Input: part model. Units: mm. Frame: model coordinates. A direction names the side the tool comes from. Give positions to 0.01 mm unless a question says otherwise; leave off trailing zeros. Write each loop counter-clockwise with the first axis right and the second up, starting at its lowest first coordinate (ties: lowest second). Pieces come first, ordered by that corner, then holes. Notation, with made-up numbers: (83, 49.5) -> (136, 49.5) arc R32 ccw to (136, 76.5) -> close; hole circle Ø1 at (-34, 74). An arc over 180 degrees is marked (long way). Answer as a JSON object with one key per item and string values. Group by question number.
from build123d import *

# Parameters (mm, degrees)
F0_R     = 30
F0_W     = 4
F0_H     = 4
F0_R_2   = 1.5
F1_DEPTH = 4
F2_R     = 2.25
F3_DEPTH = 2.6
F4_R     = 19
F4_R_2   = 1.5
F5_DEPTH = 0.1


with BuildPart() as f1:
    # F0 (on Top) → F1 (new body)
    with BuildSketch(Plane.XY):
        Circle(F0_R)
        with Locations((-26, 0)):
            Rectangle(F0_W, F0_H, mode=Mode.SUBTRACT)
        Circle(F0_R_2, mode=Mode.SUBTRACT)
        with Locations((26, 0)):
            Rectangle(F0_W, F0_H, mode=Mode.SUBTRACT)
    extrude(amount=F1_DEPTH)

    # F2 (on face) → F3 (cut)
    with BuildSketch(Plane.XY.offset(4)):
        with Locations((-18.197132, 18.083166)):
            Circle(F2_R)
        with Locations((18.083166, 18.197132)):
            Circle(F2_R)
        with Locations((-18.083166, -18.197132)):
            Circle(F2_R)
        with Locations((18.197132, -18.083166)):
            Circle(F2_R)
    extrude(amount=-F3_DEPTH, mode=Mode.SUBTRACT)

    # F4 (on face) → F5 (cut)
    with BuildSketch(Plane.XY.offset(4)):
        Circle(F4_R)
        Circle(F4_R_2, mode=Mode.SUBTRACT)
    extrude(amount=-F5_DEPTH, mode=Mode.SUBTRACT)


solid = f1.part
1. Section B-B (x = 0). Return the cut outline in (y, z), plus the area to 4 significant figures.
2. Section D-D (x = 10). Return the cut outline in (y, z).
3. Line query: line 1 (Y direction, x = 0, z = 3); line 2 (Y direction, x = 0, z = 3.95); line 3 (Z direction, x = -2.5, y = 4.5). Output: solid intervals per line, ascending.
4. Section C-C (z = 2.55). Return the cut outline in (x, y), plus the area to 3 significant figures.
5. Section A-A (y = 0). Return the cut outline in (x, z).
6. Contact query for flat-ended pins moving along their axis: pin 1 Ø1.3 at (x, y) = (-17.5, -17.5) entering from +Z; pin 2 Ø2.5 at (x, y) = (0, 0) entering from -Z; pin 3 Ø1 at (x, z) = (10.5, 3.5) entering from +Y; pin 4 Ø1.2 at (x, z) = (25, 2) entering from +Y. Output: stop coordinate, or through.
7. Reachability of faces 1 (the face through (28, 0, 2)), 2 (the face through (6, 0, 0)), 3 (the face through (-17.04, -20.19, 2.72)) from +Z, -Z, +X, -X, +Y, -Y: full face, straight path, thin tool, end or side. Return the list, or none.
Working result:
{
 "1": {"outline": "(-30, 0) -> (-1.5, 0) -> (-1.5, 3.9) -> (-19, 3.9) -> (-19, 4) -> (-30, 4) -> close; (1.5, 0) -> (30, 0) -> (30, 4) -> (19, 4) -> (19, 3.9) -> (1.5, 3.9) -> close", "area": "224.5 mm^2"},
 "2": {"outline": "(-28.28, 0) -> (28.28, 0) -> (28.28, 4) -> (16.16, 4) -> (16.16, 3.9) -> (-16.16, 3.9) -> (-16.16, 4) -> (-28.28, 4) -> close"},
 "3": {"line 1": "y = -30 to -1.5, 1.5 to 30", "line 2": "y = -30 to -19, 19 to 30", "line 3": "z = 0 to 3.9"},
 "4": {"outline": "circle Ø60 at (0, 0); hole (-28, -2) -> (-24, -2) -> (-24, 2) -> (-28, 2) -> close; hole circle Ø4.5 at (-18.2, 18.08); hole circle Ø4.5 at (-18.08, -18.2); hole circle Ø3 at (0, 0); hole circle Ø4.5 at (18.08, 18.2); hole circle Ø4.5 at (18.2, -18.08); hole (24, -2) -> (28, -2) -> (28, 2) -> (24, 2) -> close", "area": "2,720 mm^2"},
 "5": {"outline": "(-30, 0) -> (-28, 0) -> (-28, 4) -> (-30, 4) -> close; (-24, 0) -> (-1.5, 0) -> (-1.5, 3.9) -> (-19, 3.9) -> (-19, 4) -> (-24, 4) -> close; (1.5, 0) -> (24, 0) -> (24, 4) -> (19, 4) -> (19, 3.9) -> (1.5, 3.9) -> close; (28, 0) -> (30, 0) -> (30, 4) -> (28, 4) -> close"},
 "6": {"pin 1": "stops at z = 1.4", "pin 2": "passes through", "pin 3": "stops at y = 28.28", "pin 4": "stops at y = 17.45"},
 "7": {"face 1": "+Z, -Z", "face 2": "-Z, +X, -X, +Y, -Y", "face 3": "+Z"}
}
